Here's how the part is built. I have some questions about the finished solid (model axes, mm). Coordinates: 2 decimals unless noted, no trailing zeros. Loops run counter-clockwise (first coordinate to the right, second up) from the corner with the lowest first, then second, coordinate; pieces in that order, holes last. Notation, with made-up numbers: (-36.5, 29.25) - (-6.5, 29.25) arc R15 cw to (-6.5, 55.25) - close; hole circle Ø4 at (47, 53.25). An arc over 180 degrees is marked (long way). Use a Markdown table: item, result.
Autodesk Inventor part; units mm, degrees
ref_plane "YZ Plane" through (0, 0, 0) normal (1, 0, 0) x (0, 1, 0)
ref_plane "XZ Plane" through (0, 0, 0) normal (0, 1, 0) x (-1, 0, 0)
ref_plane "XY Plane" through (0, 0, 0) normal (0, 0, 1) x (1, 0, 0)
sketch "Эскиз1" plane through (0, 0, 0) normal (0, 0, 1) x (1, 0, 0)
  line L0 (0, 0) -> (37.7119, 0)
  line L1 (0, 22.5) -> (30, 22.5)
  line L2 (0, 30) -> (30, 30)
  line L3 (0, 30) -> (0, 22.5)
  line L4 (30, 30) -> (30, 22.5)
  dimension "d0" = 45
  dimension "d1" = 30
  dimension "d3" = 60
revolve "Вращение1" add sketch "Эскиз1" angle 360 about axis through (0, 0, 0) along (1, 0, 0)
chamfer "Фаска1" distance 0.7 angle 45 4 edges at (30, -30, 0) (30, -22.5, 0) (0, -22.5, 0) (0, -30, 0)
properties part number "Скольжение"
Q1. If we mould it in two halves opening along Y, with no side actions, what happens to faces 1 (the face through (15.2, -29.97, 1.32)), 2 (the face through (15.2, 10.382, -19.961)), 3 (the face through (0, -9, 22))? For each: pulls with the +Y half, pulls with the -Y half, needs draft (parallel to the pull), parting line crosses it, or undercut.
Check values:
| item | result |
|---|---|
| face 1 | parting line crosses it |
| face 2 | undercut |
| face 3 | needs draft |
Q2. I want a section at A-A, the plane y = 0. Write out the boundary of the cut face in (x, z), then the cut area to 3 significant figures.
Check values:
| item | result |
|---|---|
| outline | (0, -29.3) - (0.7, -30) - (29.3, -30) - (30, -29.3) - (30, -23.2) - (29.3, -22.5) - (0.7, -22.5) - (0, -23.2) - close; (0, 23.2) - (0.7, 22.5) - (29.3, 22.5) - (30, 23.2) - (30, 29.3) - (29.3, 30) - (0.7, 30) - (0, 29.3) - close |
| area | 448 mm^2 |
Q3. I want a section at C-C, the plane x = 2.5. Write out the boundary of the cut face in (y, z), then the cut area to 3 significant figures.
Check values:
| item | result |
|---|---|
| outline | circle Ø60 at (0, 0); hole circle Ø45 at (0, 0) |
| area | 1,240 mm^2 |
Q4. Please list where these lines run through material, in increasing order: L1, parallel to Z at x = 20.75, y = 0; L2, parallel to Y at x = 24.5, z = 9.5; L3, parallel to Y at x = 5.25, z = -12.5. Write a range as from..to.
Check values:
| item | result |
|---|---|
| L1 | -30..-22.5, 22.5..30 |
| L2 | -28.46..-20.4, 20.4..28.46 |
| L3 | -27.27..-18.71, 18.71..27.27 |
Q5. Will these pins go through, and if not, where does the flat tip stop? P1, Ø4, axis at x = 22.5, y = -13, coming from the +Z side; P2, Ø4, axis at x = 3, y = -11.5, coming from the -Z side; P3, Ø10, axis at x = 9, z = 6.5, coming from the +Y side; P4, Ø12, axis at y = 5.5, z = 15, coming from the -X side.
Check values:
| item | result |
|---|---|
| P1 | z = 27.91 |
| P2 | z = -28.46 |
| P3 | y = 29.96 |
| P4 | through |
